Here's the drawing with two shaded views (mm, measured from the low corner). I have some questions. A direction names the side the tool comes from. Give positions to 0.01 mm unless a question says otherwise; leave off trailing zeros. Order: outer loops, then holes, each group sorted by start corner. A loop starts at its lowest first (then second) coordinate and runs counter-clockwise, first axis right, second up. Notation, with made-up numbers: (-29.5, 56.5) - (16.5, 56.5) arc R25 cw to (16.5, 74.5) - close; hole circle Ø5 at (58.5, 89). An arc over 180 degrees is marked (long way). Use one line per item in the form item = value. Start each with the question number.
1) Suppose I cut it at B-B, the plane z = 11. Write out the boundary of the cut face in (x, y), and give its area (3 significant figures).
2) Please list where these lines run through material, in increasing order: probe 1 along Y at (x, z) = (45, 21.5); probe 2 along X at (y, z) = (6, 29); probe 3 along Z at (x, y) = (16, 3).
3) For pin 1 (1.5 mm diameter, centred on x = 13, y = 1.5, fed in from +Z); pin 2 (1.5 mm diameter, centred on y = 38, z = 42.5, fed in from -X); pin 3 (3 mm diameter, centred on x = 34, z = 37, fed in from -Y); pin 4 (1.5 mm diameter, centred on x = 6.5, y = 18.5, fed in from +Z), each with a flat end and sliding along its axis, tell me the tip position at first contact or that it passes through.
4) Suppose I cut it at A-A, the plane y = 16. Write out the boundary of the cut face in (x, z).
5) Suppose I cut it at C-C, the plane x = 8. Write out the boundary of the cut face in (y, z), and give its area (3 significant figures).
6) Which directions (+Z, -Z, +X, -X, +Y, -Y) give clear straight access to the entire face, cutting with the end or side of a thin tool? Please do the marked faces 5 and 6.
7) We'd pull the mould along X, two halves only. Please class the marked faces 1, 2, 3 and 4: released by +X, released by -X, zero draft, split by the parting line, or undercut.
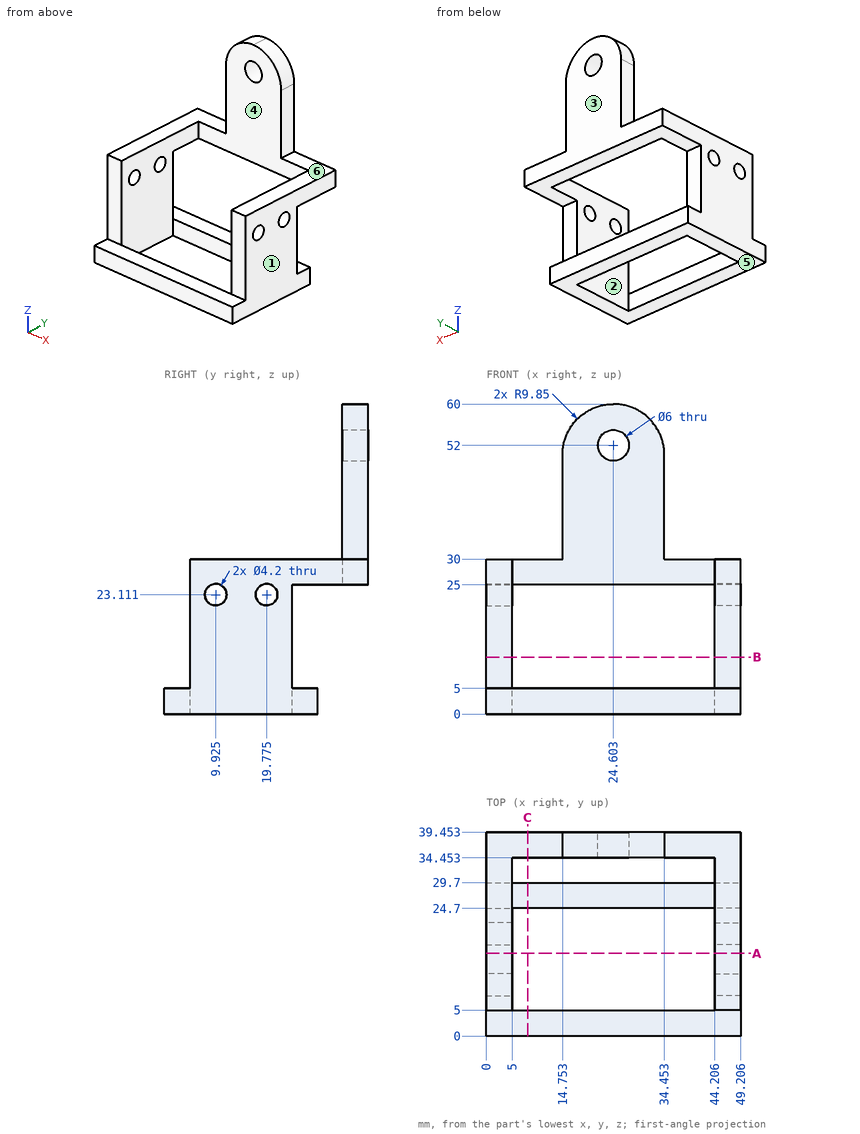
Result sheet:
q1.outline = (0, 5) - (5, 5) - (5, 24.7) - (0, 24.7) - close; (44.21, 5) - (49.21, 5) - (49.21, 24.7) - (44.21, 24.7) - close
q1.area = 197 mm²
q2.probe_1 = 5 to 8.58, 11.27 to 18.43, 21.12 to 24.7
q2.probe_2 = 0 to 5, 44.21 to 49.21
q2.probe_3 = 0 to 5
q3.pin_1 = 5
q3.pin_2 = 14.75
q3.pin_3 = 34.45
q3.pin_4 = through
q4.outline = (0, 0) - (5, 0) - (5, 30) - (0, 30) - close; (44.21, 0) - (49.21, 0) - (49.21, 30) - (44.21, 30) - close
q5.outline = (0, 0) - (5, 0) - (5, 5) - (0, 5) - close; (24.7, 0) - (29.7, 0) - (29.7, 5) - (24.7, 5) - close; (34.45, 25) - (39.45, 25) - (39.45, 30) - (34.45, 30) - close
q5.area = 75.0 mm²
q6.face_5 = -Z, +X, -X, +Y, -Y
q6.face_6 = +Z, +X, +Y, -Y
q7.face_1 = released by +X
q7.face_2 = undercut
q7.face_3 = zero draft
q7.face_4 = undercut
